from build123d import *

# Parameters (mm, degrees)
SKETCH1_R           = 11.5
SKETCH1_R_2         = 8.5
BOSS_EXTRUDE1_DEPTH = 0.4
SKETCH2_R           = 0.6
BOSS_EXTRUDE2_DEPTH = 1
SKETCH3_R           = 0.5
BOSS_EXTRUDE3_DEPTH = 1
CUT_EXTRUDE1_START  = -0.4
CUT_EXTRUDE1_DEPTH  = 0.4
DRAFT2_ANGLE        = -1


with BuildPart() as part:
    # Sketch1 → Boss-Extrude1 (new body)
    with BuildSketch(Plane(origin=(0, 0, 0), x_dir=(1, 0, 0), z_dir=(0, 1, 0))):
        with Locations(Location((0, 1.53064501, 0), (0, 0, 270))):
            Circle(SKETCH1_R)
        with Locations(Location((0, 1.53064501, 0), (0, 0, 270))):
            Circle(SKETCH1_R_2, mode=Mode.SUBTRACT)
    extrude(amount=BOSS_EXTRUDE1_DEPTH)

    # Sketch2 → Boss-Extrude2 (add)
    with BuildSketch(Plane(origin=(0, 0, 0), x_dir=(1, 0, 0), z_dir=(0, 1, 0))):
        with Locations(Location((-4.61588, -8.175151, 0), (0, 0, 270))):
            Circle(SKETCH2_R)
        with Locations(Location((-7.04588, 8.574849, 0), (0, 0, 270))):
            Circle(SKETCH2_R)
        with Locations(Location((7.74412, 8.574849, 0), (0, 0, 90))):
            Circle(SKETCH2_R)
        with Locations(Location((4.45412, -8.175151, 0), (0, 0, 90))):
            Circle(SKETCH2_R)
    extrude(amount=-BOSS_EXTRUDE2_DEPTH)

    # Sketch3 → Boss-Extrude3 (add)
    with BuildSketch(Plane.XZ.offset(1)):
        with Locations(Location((-4.61588, 8.175151, 0), (0, 0, 270))):
            Circle(SKETCH3_R)
        with Locations(Location((-7.04588, -8.574849, 0), (0, 0, 270))):
            Circle(SKETCH3_R)
        with Locations(Location((7.74412, -8.574849, 0), (0, 0, 90))):
            Circle(SKETCH3_R)
        with Locations(Location((4.45412, 8.175151, 0), (0, 0, 90))):
            Circle(SKETCH3_R)
    extrude(amount=BOSS_EXTRUDE3_DEPTH)

    # Sketch6 → Cut-Extrude1 (cut)
    with BuildSketch(Plane(origin=(0, 0.4, 0), x_dir=(1, 0, 0), z_dir=(0, 1, 0)).offset(CUT_EXTRUDE1_START)):
        with BuildLine():
            Line((3, -9), (-3, -9))
            Line((-3, -9), (-3, -9.571156646))
            ThreePointArc((-3, -9.571156646), (0, -9.96935499), (3, -9.571156646))
            Line((3, -9.571156646), (3, -9))
        make_face()
    extrude(amount=CUT_EXTRUDE1_DEPTH, mode=Mode.SUBTRACT)

    # Draft2
    draft2_faces = [part.faces().sort_by_distance(p)[0] for p in [
        (7.74412, -1.5, -9.074849),
        (7.74412, -0.5, -7.974849),
        (4.45412, -0.5, 8.775151),
        (4.45412, -1.5, 7.675151),
        (-4.61588, -1.5, 8.675151),
        (-4.61588, -0.5, 7.575151),
        (-7.04588, -0.5, -9.174849),
        (-7.04588, -1.5, -8.074849),
    ]]
    draft(draft2_faces, Plane.ZX, DRAFT2_ANGLE)


solid = part.part
Geometry check sheet. Reference: the model listing, model coordinates, mm. A direction names the side the tool comes from. Round coordinates to 2 decimals unless told otherwise and drop trailing zeros. Loops run counter-clockwise (first coordinate to the right, second up) from the corner with the lowest first, then second, coordinate; pieces in that order, holes last. Notation, with made-up numbers: (75.5, 77) - (126.5, 77) arc R22 ccw to (126.5, 109) - close; hole circle Ø7 at (-14, -8.75). An arc over 180 degrees is marked (long way). Answer as CSV lines item,"result".
(1) Cross-section at D-D, the plane x = 9.5. Enter the section's corners in (y, z).
Output values:
outline,"(0, -8.01) - (0.4, -8.01) - (0.4, 4.95) - (0, 4.95) - close"
(2) Cross-section at C-C, the plane y = -0.4. Enter the section's corners in (x, z), and give its area (3 significant figures).
Output values:
outline,"circle Ø1.19 at (-7.05, -8.57); circle Ø1.19 at (-4.62, 8.18); circle Ø1.19 at (4.45, 8.18); circle Ø1.19 at (7.74, -8.57)"
area,"4.42 mm²"
(3) Cross-section at B-B, the plane z = -0.5. Enter the section's corners in (x, y).
Output values:
outline,"(-11.45, 0) - (-8.44, 0) - (-8.44, 0.4) - (-11.45, 0.4) - close; (8.44, 0) - (11.45, 0) - (11.45, 0.4) - (8.44, 0.4) - close"
(4) Set-up check for faces 1 (the face through (-7.334, -1.493, -8.199)), 2 (the face through (0.9, 0.4, -10.2)): record each of +Z, -Z, +X, -X, +Y, -Y from which the full face is reachable in a straight line by a thin tool's end or side.
Output values:
face 1,"-Y"
face 2,"+Z, -Z, +X, -X, +Y"
(5) Release check for a two-part mould opening along X. For faces 3 (the face through (-4.59, -0.493, 7.584)), 4 (the face through (0.46, 0.2, -13.02)), 5 (the face through (-4.6, -2, 8.2)), 6 (the face through (8.033, -1.493, -8.951)) record: released by +X, released by -X, zero draft, split by the parting line, or undercut.
Output values:
face 3,"undercut"
face 4,"split by the parting line"
face 5,"zero draft"
face 6,"undercut"
(6) Material ranges on line 1 along Y through (x, z) = (-5.5, 5); line 2 along Z through (x, y) = (2.5, 0.05); line 3 along X through (y, z) = (0.1, 1), recorded low to high.
Output values:
line 1,"y = 0 to 0.4"
line 2,"z = -12.76 to -9.65, 6.59 to 9"
line 3,"x = -11.22 to -8.11, 8.11 to 11.22"
(7) Depth check by flat-ended pin: pin 1 Ø11.5 at (x, z) = (-5, -2.5) entering from -Y. Enter the tip coordinate at first touch or a pass-through.
Output values:
pin 1,"stops at y = 0"
(8) Cross-section at A-A, the plane x = 0. Enter the section's corners in (y, z), and give its area (3 significant figures).
Output values:
outline,"(0, -13.03) - (0.4, -13.03) - (0.4, -10.03) - (0, -10.03) - close; (0, 6.97) - (0.4, 6.97) - (0.4, 9) - (0, 9) - close"
area,"2.01 mm²"
